Here's how the part is built. I have some questions about the finished solid (model axes, mm). A direction names the side the tool comes from. Give positions to 0.01 mm unless a question says otherwise; leave off trailing zeros. Order: outer loops, then holes, each group sorted by start corner. A loop starts at its lowest first (then second) coordinate and runs counter-clockwise, first axis right, second up. Notation, with made-up numbers: (71, 78.5) - (101, 78.5) arc R20 ccw to (101, 87.5) - close; hole circle Ø10 at (4, 20.5). An arc over 180 degrees is marked (long way). One line per question, with ' | ' between items.
from build123d import *

# Parameters (mm, degrees)
SKETCH1_W            = 40
SKETCH1_H            = 100
BOSS_EXTRUDE1_DEPTH  = 3
FILLET1_R            = 20
SKETCH2_W            = 40
SKETCH2_H            = 10
BOSS_EXTRUDE2_DEPTH  = 27
M3_CLEARANCE_HOLE1_D = 3.4
BOSS_EXTRUDE4_DEPTH  = 3


with BuildPart() as part:
    # Sketch1 → Boss-Extrude1 (new body)
    with BuildSketch(Plane.XY):
        with Locations((20, 24.444444444)):
            Rectangle(SKETCH1_W, SKETCH1_H)
    extrude(amount=BOSS_EXTRUDE1_DEPTH)

    # Fillet1
    fillet1_edges = [part.edges().sort_by_distance(p)[0] for p in [
        (40, -25.555555556, 1.5),
        (0, -25.555555556, 1.5),
    ]]
    fillet(fillet1_edges, radius=FILLET1_R - 0.0001)  # a hair under: the kernel refuses the full size

    # Sketch2 → Boss-Extrude2 (add)
    with BuildSketch(Plane(origin=(0, 0, 0), x_dir=(-1, 0, 0), z_dir=(0, 0, -1))):
        with Locations((-20, 69.444444444)):
            Rectangle(SKETCH2_W, SKETCH2_H)
    extrude(amount=BOSS_EXTRUDE2_DEPTH)

    # M3 Clearance Hole1 (through all)
    with Locations(Plane(origin=(0, 64.444444444, 0), x_dir=(-1, 0, 0), z_dir=(0, -1, 0))):
        with Locations((-28.8, 6.190883488), (-11.2, 6.190883488)):
            Hole(M3_CLEARANCE_HOLE1_D / 2)

    # Sketch15 → Boss-Extrude4 (add)
    with BuildSketch(Plane.XY.offset(3)):
        with BuildLine():
            Line((85, 74.444444444), (40, 74.444444444))
            Line((40, 74.444444444), (40, 29.444444444))
            ThreePointArc((40, 29.444444444), (56.606100623, 57.838343821), (85, 74.444444444))
        make_face()
        with BuildLine():
            Line((0, 29.444444444), (0, 74.444444444))
            Line((0, 74.444444444), (-45, 74.444444444))
            ThreePointArc((-45, 74.444444444), (-16.606100623, 57.838343821), (0, 29.444444444))
        make_face()
    extrude(amount=-BOSS_EXTRUDE4_DEPTH)


solid = part.part
1) Thinking about a two-plate mould opening in Z: for faces 1 (the face through (21, 74.444, -8)), 2 (the face through (19, 36, 3)), 3 (the face through (9.85, 69.51, -5.16)), which applies, +Z half, -Z half, draft (parallel to the pull), parting line (faces both ways), or undercut?
Model answer:
face 1: draft | face 2: +Z half | face 3: undercut
2) I want a section at B-B (y = 26). List the corners of the cut face in (x, z) for me.
Model answer:
outline: (0, 0) - (40, 0) - (40, 3) - (0, 3) - close
3) I want a section at A-A (x = 28.8). List the corners of the cut face in (y, z) for me.
Model answer:
outline: (-23.52, 0) - (64.44, 0) - (64.44, -4.49) - (74.44, -4.49) - (74.44, 3) - (-23.52, 3) - close; (64.44, -27) - (74.44, -27) - (74.44, -7.89) - (64.44, -7.89) - close
4) Please list where these lines run through material, in increasing order: L1, parallel to Z at x = 11.2, y = 70.5; L2, parallel to Y at x = 28, z = -10.5; L3, parallel to Z at x = 32, y = 40.5.
Model answer:
L1: z = -27 to -7.89, -4.49 to 3 | L2: y = 64.44 to 74.44 | L3: z = 0 to 3
5) I want a section at C-C (z = -14.25). List the corners of the cut face in (x, y) for me.
Model answer:
outline: (0, 64.44) - (40, 64.44) - (40, 74.44) - (0, 74.44) - close
6) On a 3-axis mill with a long thin cutter (end or side, diameter ignored), from which of +Z, -Z, +X, -X, +Y, -Y can I reach the whole of each face in a straight line? I mean faces 4 (the face through (0, 12, 2)), 5 (the face through (40, 69, -13)), 6 (the face through (20, 64.444, -13)), 7 (the face through (40, 12, 2)). Say none if no direction works.
Model answer:
face 4: +Z, -Z, -X, -Y | face 5: -Z, +X, +Y, -Y | face 6: -Z, +X, -X, -Y | face 7: +Z, -Z, +X, -Y
7) I'm going to push flat-ended pins straight in: P1, Ø10, axis at x = -0.5, z = -18.5, coming from the -Y side; P2, Ø3.5, axis at y = 12.5, z = 1, coming from the +X side; P3, Ø5, axis at y = 67, z = -14, coming from the -X side; P4, Ø12, axis at y = 57, z = -20.5, coming from the +X side. Where does each tip first touch, or does it pass through?
Model answer:
P1: stops at y = 64.44 | P2: stops at x = 40 | P3: stops at x = 0 | P4: passes through
